```python
from build123d import *

# Parameters (mm, degrees)
BOSS_EXTRUDE1_DEPTH = 40
FILLET1_R           = 0.8


with BuildPart() as part:
    # Sketch1 → Boss-Extrude1 (new body)
    with BuildSketch(Plane.XY):
        Polygon((0, 0), (21.1, 0), (21.1, 1.6), (19.5, 1.6), (19.5, 0.8), (0, 0.8), align=None)
    extrude(amount=BOSS_EXTRUDE1_DEPTH)

    # Fillet1
    fillet1_edges = [part.edges().sort_by_distance(p)[0] for p in [
        (19.5, 1.2, 0),
        (0, 0.4, 0),
        (21.1, 0.8, 0),
        (19.5, 1.2, 40),
        (21.1, 0.8, 40),
        (0, 0.4, 40),
    ]]
    fillet(fillet1_edges, radius=FILLET1_R - 0.0001)  # a hair under: the kernel refuses the full size


solid = part.part
```
Could you check a few things on this model? Use its own coordinates, in mm. Round coordinates to 2 decimals unless told otherwise and drop trailing zeros. Loops run counter-clockwise (first coordinate to the right, second up) from the corner with the lowest first, then second, coordinate; pieces in that order, holes last.
Q1. I want a section at A-A (z = 34). Write out the boundary of the cut face in (x, y).
Q2. I want a section at C-C (x = 7.25). Write out the boundary of the cut face in (y, z).
Q3. For P1, Ø1.5, axis at x = 11.5, z = 32.5, coming from the +Y side, with a flat end and sliding along its axis, tell me the tip position at first contact or that it passes through.
Q4. Please list where these lines run through material, in increasing order: L1, parallel to Y at x = 11, z = 24.5; L2, parallel to X at y = 1.25, z = 4.
Answer below:
1. outline: (0, 0) - (21.1, 0) - (21.1, 1.6) - (19.5, 1.6) - (19.5, 0.8) - (0, 0.8) - close
2. outline: (0, 0) - (0.8, 0) - (0.8, 40) - (0, 40) - close
3. P1: stops at y = 0.8
4. L1: y = 0 to 0.8
4. L2: x = 19.5 to 21.1
